from build123d import *

# Parameters (mm, degrees)
CROQUIS1_R              = 3.75
CROQUIS1_W              = 3
CROQUIS1_H              = 12.3
SALIENTE_EXTRUIR1_DEPTH = 3


with BuildPart() as part:
    # Croquis1 → Saliente-Extruir1 (new body)
    with BuildSketch(Plane.XY):
        Polygon((-34.033695548, 97.071783877), (-101.583677043, 58.071783877), (-101.583677043, -19.928216123), (-34.033695548, -58.928216123), (33.516285947, -19.928216123), (33.516285947, 58.071783877), align=None)
        with Locations((-90.325346794, 47.821783877)):
            Circle(CROQUIS1_R, mode=Mode.SUBTRACT)
        Polygon((-51.384514513, 1.319283877), (-52.884514513, -1.278792335), (-42.232402047, -7.428792335), (-40.732402047, -4.830716123), align=None, mode=Mode.SUBTRACT)
        Polygon((-26.461178531, 83.163890705), (-27.949867087, 80.559283877), (-17.297738084, 74.409274329), (-15.809049529, 77.013881158), align=None, mode=Mode.SUBTRACT)
        Polygon((7.033309637, 63.825838945), (17.685438639, 57.675829398), (16.174127236, 55.084283877), (5.521998234, 61.234293424), align=None, mode=Mode.SUBTRACT)
        Polygon((5.521998234, -23.090725671), (7.033309637, -25.682271192), (17.685438639, -19.532261645), (16.174127236, -16.940716123), align=None, mode=Mode.SUBTRACT)
        Polygon((-9.725254139, 73.501400252), (-11.213942694, 70.896793424), (-0.561813692, 64.746783877), (0.926874864, 67.351390705), align=None, mode=Mode.SUBTRACT)
        Polygon((0.926874864, -29.207822952), (-9.725254139, -35.357832499), (-11.213942694, -32.753225671), (-0.561813692, -26.603216123), align=None, mode=Mode.SUBTRACT)
        Polygon((-15.809049529, -38.870313405), (-26.461178531, -45.020322952), (-27.949867087, -42.415716123), (-17.297738084, -36.265706576), align=None, mode=Mode.SUBTRACT)
        Polygon((-50.769653012, -36.265706576), (-52.258341568, -38.870313405), (-41.606212565, -45.020322952), (-40.11752401, -42.415716123), align=None, mode=Mode.SUBTRACT)
        Polygon((-67.505577405, -26.603216123), (-68.99426596, -29.207822952), (-58.342136958, -35.357832499), (-56.853448402, -32.753225671), align=None, mode=Mode.SUBTRACT)
        Polygon((-84.241518333, -16.940716123), (-73.58938933, -23.090725671), (-75.100700733, -25.682271192), (-85.752829736, -19.532261645), align=None, mode=Mode.SUBTRACT)
        Polygon((-73.58938933, 61.234293424), (-75.100700733, 63.825838945), (-85.752829736, 57.675829398), (-84.241518333, 55.084283877), align=None, mode=Mode.SUBTRACT)
        Polygon((-68.99426596, 67.351390705), (-58.342136958, 73.501400252), (-56.853448402, 70.896793424), (-67.505577405, 64.746783877), align=None, mode=Mode.SUBTRACT)
        Polygon((-52.258341568, 77.013881158), (-41.606212565, 83.163890705), (-40.11752401, 80.559283877), (-50.769653012, 74.409274329), align=None, mode=Mode.SUBTRACT)
        with Locations((23.757955698, 38.396783877)):
            Rectangle(CROQUIS1_W, CROQUIS1_H, mode=Mode.SUBTRACT)
        with Locations((23.757955698, 19.071783877)):
            Rectangle(CROQUIS1_W, CROQUIS1_H, mode=Mode.SUBTRACT)
        with Locations((23.757955698, -0.253216123)):
            Rectangle(CROQUIS1_W, CROQUIS1_H, mode=Mode.SUBTRACT)
        Polygon((-25.83498905, 45.572360088), (-15.182876583, 39.422360088), (-16.682876583, 36.824283877), (-27.33498905, 42.974283877), align=None, mode=Mode.SUBTRACT)
        Polygon((-52.884514513, 39.422360088), (-42.232402047, 45.572360088), (-40.732402047, 42.974283877), (-51.384514513, 36.824283877), align=None, mode=Mode.SUBTRACT)
        Polygon((-27.33498905, -4.830716123), (-25.83498905, -7.428792335), (-15.182876583, -1.278792335), (-16.682876583, 1.319283877), align=None, mode=Mode.SUBTRACT)
        with Locations((-8.484170085, 19.071783877)):
            Rectangle(CROQUIS1_W, CROQUIS1_H, mode=Mode.SUBTRACT)
        with Locations((-59.583221011, 19.071783877)):
            Rectangle(CROQUIS1_W, CROQUIS1_H, mode=Mode.SUBTRACT)
    extrude(amount=SALIENTE_EXTRUIR1_DEPTH)


solid = part.part
Check sheet for the modelled part. Datum: model origin and axes. Units: mm. Give positions to 0.01 mm unless a question says otherwise; leave off trailing zeros. Write each loop counter-clockwise with the first axis right and the second up, starting at its lowest first coordinate (ties: lowest second). Pieces come first, ordered by that corner, then holes. Notation, with made-up numbers: (84.5, 42) -> (116.5, 42) arc R27 ccw to (116.5, 80) -> close; hole circle Ø11 at (80.5, 84.25). An arc over 180 degrees is marked (long way). One line per item, written item: value. Start each with the question number.
Item 1: Material ranges on probe 1 along X at (y, z) = (15, 1.45); probe 2 along Y at (x, z) = (-68, 1); probe 3 along X at (y, z) = (77.5, 1.7), recorded low to high. Write a range as from..to.
Item 2: Section check B-B on x = -44. Record the cut outline in (y, z).
Item 3: Section check C-C on z = 2.05. State how many separate pieces and enclosed holes the cut face has, then the cut area to 3 significant figures.
Item 4: Gauge pin test, flat ends, axial feed: pin 1 (1 mm diameter, centred on x = -14, z = 1.5, fed in from -Y); pin 2 (1.5 mm diameter, centred on x = -8, z = 1, fed in from -Y); pin 3 (1.5 mm diameter, centred on x = 24.5, z = 1.5, fed in from +Y). Record the tip position at first contact, or that the pin passes through.
Item 5: Section check A-A on y = 20.5. Record the cut outline in (x, z), then the cut area to 3 significant figures.
Item 6: Draft check along X on faces 1 (the flat face through (-35, 20, 0)), 2 (the flat face through (-67.336, 77.845, 1.479)), 3 (the flat face through (-45.369, -39.384, 1.479)). Enter one of: +X half, -X half, draft (parallel to the pull), parting line (faces both ways), or undercut.
Results list:
1. probe 1: -101.58..-61.08, -58.08..-9.98, -6.98..22.26, 25.26..33.52
1. probe 2: -39.32..-29.78, -27.47..65.61, 67.93..77.46
1. probe 3: -67.93..-51.42, -45.42..-22.65, -16.65..-0.13
2. outline: (-53.17, 0) -> (-43.64, 0) -> (-43.64, 3) -> (-53.17, 3) -> close; (-40.17, 0) -> (-6.41, 0) -> (-6.41, 3) -> (-40.17, 3) -> close; (-2.94, 0) -> (41.09, 0) -> (41.09, 3) -> (-2.94, 3) -> close; (44.55, 0) -> (78.32, 0) -> (78.32, 3) -> (44.55, 3) -> close; (81.78, 0) -> (91.32, 0) -> (91.32, 3) -> (81.78, 3) -> close
3. separate pieces: 1
3. enclosed holes: 22
3. area: 15,000 mm²
4. pin 1: y = -47.65
4. pin 2: y = -44.33
4. pin 3: y = 63.71
5. outline: (-101.58, 0) -> (-61.08, 0) -> (-61.08, 3) -> (-101.58, 3) -> close; (-58.08, 0) -> (-9.98, 0) -> (-9.98, 3) -> (-58.08, 3) -> close; (-6.98, 0) -> (22.26, 0) -> (22.26, 3) -> (-6.98, 3) -> close; (25.26, 0) -> (33.52, 0) -> (33.52, 3) -> (25.26, 3) -> close
5. area: 378 mm²
6. face 1: draft
6. face 2: -X half
6. face 3: undercut
